Work out the finished part from the listing and answer in its coordinate system (mm). Face numbers are marked on the shaded views. A direction names the side the tool comes from. Give positions to 0.01 mm unless a question says otherwise; leave off trailing zeros. Write each loop counter-clockwise with the first axis right and the second up, starting at its lowest first coordinate (ties: lowest second). Pieces come first, ordered by that corner, then holes.
1) Given pin 1 Ø2 at (y, z) = (-7, 47) entering from +X; pin 2 Ø12 at (x, y) = (37, 0) entering from -Z; pin 3 Ø8.5 at (x, y) = (130.58, -8.08) entering from +Z; pin 4 Ø6 at (y, z) = (-6, 15) entering from -X, each flat-ended and moving along its own axis, determine where each tip first touches the part or whether it passes through.
2) Find section D-D (x = -1.5). Determine the outline of the cut face in (y, z), plus the area to 3 significant figures.
3) A tool of negligible diameter and unlimited length cuts with its end or side. For the marked faces 5, 6, 7 and 8, from which of +Z, -Z, +X, -X, +Y, -Y can it reach the whole face along a straight path? Write none if from no direction.
4) Find section C-C (x = 62). Determine the outline of the cut face in (y, z), plus the area to 3 significant figures.
5) Determine the mould class of the marked faces 1, 2, 3 and 4 for opening direction Z: pulls with the +Z half, pulls with the -Z half, needs draft (parallel to the pull), parting line crosses it, or undercut.
6) Find section A-A (z = 15.5). Determine the outline of the cut face in (x, y).
7) Find section B-B (y = -14). Determine the outline of the cut face in (x, z).
8) Straight lines are drawn through the part: probe 1 along X at (y, z) = (-4, 19.5); probe 2 along Z at (x, y) = (68.5, 2.5); probe 3 along Z at (x, y) = (133.5, 4). For each, find the intervals that lie inside material, in ascending order.
```python
from build123d import *

# Parameters (mm, degrees)
SKETCH1_R           = 3.175
BOSS_EXTRUDE1_DEPTH = 11.43
SKETCH2_W           = 161.464261653
SKETCH2_H           = 32
BOSS_EXTRUDE2_DEPTH = 12.7
SKETCH5_R           = 3.175
BOSS_EXTRUDE3_DEPTH = 11.43
SKETCH6_W           = 77
SKETCH6_H           = 11.5
CUT_EXTRUDE1_DEPTH  = 7.5
BOSS_EXTRUDE4_DEPTH = 19.05
CUT_EXTRUDE3_DEPTH  = 30.48
BOSS_EXTRUDE5_DEPTH = 25.4
SKETCH7_W           = 12
SKETCH7_H           = 11.5
CUT_EXTRUDE4_DEPTH  = 50.8
SKETCH7_5_W         = 12
SKETCH7_5_H         = 11.5
CUT_EXTRUDE5_DEPTH  = 50.8


with BuildPart() as part:
    # Sketch1 → Boss-Extrude1 (new body)
    with BuildSketch(Plane.XY):
        with BuildLine():
            Line((-47.217391304, 7.923913043), (130.582608696, 7.923913043))
            ThreePointArc((130.582608696, 7.923913043), (146.582608696, -8.076086957), (130.582608696, -24.076086957))
            Line((130.582608696, -24.076086957), (-47.217391304, -24.076086957))
            ThreePointArc((-47.217391304, -24.076086957), (-63.217391304, -8.076086957), (-47.217391304, 7.923913043))
        make_face()
        with Locations((-47.217391304, -8.076086957)):
            Circle(SKETCH1_R, mode=Mode.SUBTRACT)
        with Locations((130.582608696, -8.076086957)):
            Circle(SKETCH1_R, mode=Mode.SUBTRACT)
    extrude(amount=BOSS_EXTRUDE1_DEPTH)

    # Sketch2 → Boss-Extrude2 (add)
    with BuildSketch(Plane.XY.offset(11.43)):
        with Locations((41.59547787, -8.076086957)):
            Rectangle(SKETCH2_W, SKETCH2_H)
    extrude(amount=BOSS_EXTRUDE2_DEPTH)

    # Sketch5 → Boss-Extrude3 (add)
    with BuildSketch(Plane.XY.offset(24.13)):
        with BuildLine():
            Line((-47.217391304, 7.923913043), (130.582608696, 7.923913043))
            ThreePointArc((130.582608696, 7.923913043), (146.582608696, -8.076086957), (130.582608696, -24.076086957))
            Line((130.582608696, -24.076086957), (-47.217391304, -24.076086957))
            ThreePointArc((-47.217391304, -24.076086957), (-63.217391304, -8.076086957), (-47.217391304, 7.923913043))
        make_face()
        with Locations((-47.217391304, -8.076086957)):
            Circle(SKETCH5_R, mode=Mode.SUBTRACT)
        with Locations((130.582608696, -8.076086957)):
            Circle(SKETCH5_R, mode=Mode.SUBTRACT)
    extrude(amount=BOSS_EXTRUDE3_DEPTH)

    # Sketch6 → Cut-Extrude1 (cut)
    with BuildSketch(Plane(origin=(0, 7.923913043, 0), x_dir=(1, 0, 0), z_dir=(0, 1, 0))):
        with Locations((41.682608696, -17.78)):
            Rectangle(SKETCH6_W, SKETCH6_H)
    extrude(amount=-CUT_EXTRUDE1_DEPTH, mode=Mode.SUBTRACT)

    # Sketch10 → Boss-Extrude4 (add)
    with BuildSketch(Plane.XY.offset(35.56)):
        with BuildLine():
            Line((-34.517391304, -20.776086957), (-57.377391304, -20.776086957))
            ThreePointArc((-57.377391304, -20.776086957), (-59.173442529, -20.032138181), (-59.917391304, -18.236086957))
            Line((-59.917391304, -18.236086957), (-59.917391304, 2.083913043))
            ThreePointArc((-59.917391304, 2.083913043), (-59.173442529, 3.879964268), (-57.377391304, 4.623913043))
            Line((-57.377391304, 4.623913043), (-34.517391304, 4.623913043))
            Line((-34.517391304, 4.623913043), (-21.817391304, 4.623913043))
            Line((-21.817391304, 4.623913043), (-21.817391304, -20.776086957))
            Line((-21.817391304, -20.776086957), (-34.517391304, -20.776086957))
        make_face()
    extrude(amount=BOSS_EXTRUDE4_DEPTH)

    # Sketch14 → Cut-Extrude3 (cut)
    with BuildSketch(Plane(origin=(0, 4.623913043, 0), x_dir=(1, 0, 0), z_dir=(0, 1, 0))):
        with BuildLine():
            Line((-59.917391304, -35.56), (-29.183391304, -35.56))
            ThreePointArc((-29.183391304, -35.56), (-29.434604535, -44.304535578), (-35.79555952, -50.310221405))
            Line((-35.79555952, -50.310221405), (-59.917391304, -50.310221405))
            Line((-59.917391304, -50.310221405), (-59.917391304, -35.56))
        make_face()
    extrude(amount=-CUT_EXTRUDE3_DEPTH, mode=Mode.SUBTRACT)

    # Sketch15 → Boss-Extrude5 (add)
    with BuildSketch(Plane.XZ.offset(20.776086957)):
        Polygon((-21.817391304, 35.56), (5.46367495, 35.56), (-21.817391304, 54.61), align=None)
    extrude(amount=-BOSS_EXTRUDE5_DEPTH)

    # Sketch7 → Cut-Extrude4 (cut)
    with BuildSketch(Plane(origin=(0, 0.423913043, 0), x_dir=(1, 0, 0), z_dir=(0, 1, 0))):
        with Locations((74.182608696, -17.78)):
            Rectangle(SKETCH7_W, SKETCH7_H)
    extrude(amount=-CUT_EXTRUDE4_DEPTH, mode=Mode.SUBTRACT)

    # Sketch7<5> → Cut-Extrude5 (cut)
    with BuildSketch(Plane(origin=(0, 0.423913043, 0), x_dir=(1, 0, 0), z_dir=(0, 1, 0))):
        with Locations((9.182608696, -17.78)):
            Rectangle(SKETCH7_5_W, SKETCH7_5_H)
    extrude(amount=-CUT_EXTRUDE5_DEPTH, mode=Mode.SUBTRACT)


solid = part.part
```
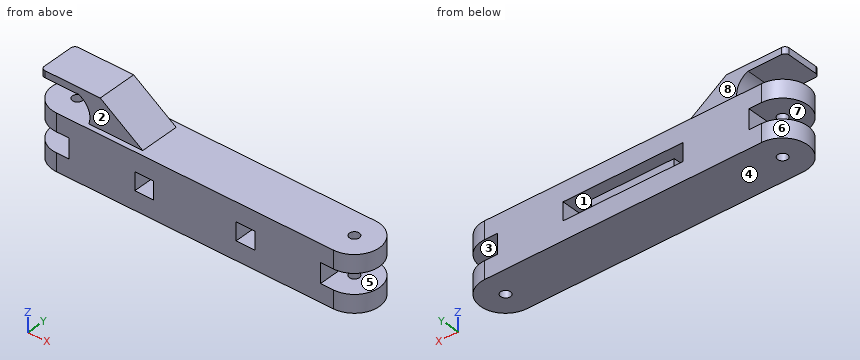
Results:
1. pin 1: stops at x = -9.49
1. pin 2: stops at z = 0
1. pin 3: stops at z = 35.56
1. pin 4: stops at x = -39.14
2. outline: (-24.08, 0) - (7.92, 0) - (7.92, 35.56) - (4.62, 35.56) - (4.62, 40.42) - (-20.78, 40.42) - (-20.78, 35.56) - (-24.08, 35.56) - close
2. area: 1,260 mm2
3. face 5: +X, +Y, -Y
3. face 6: -Z, -X
3. face 7: -X, +Y, -Y
3. face 8: +Z, +X, -X, +Y
4. outline: (-24.08, 0) - (7.92, 0) - (7.92, 12.03) - (0.42, 12.03) - (0.42, 23.53) - (7.92, 23.53) - (7.92, 35.56) - (-24.08, 35.56) - close
4. area: 1,050 mm2
5. face 1: undercut
5. face 2: needs draft
5. face 3: undercut
5. face 4: pulls with the -Z half
6. outline: (-39.14, -24.08) - (3.18, -24.08) - (3.18, 7.92) - (-39.14, 7.92) - close; (15.18, -24.08) - (68.18, -24.08) - (68.18, 0.42) - (15.18, 0.42) - close; (80.18, -24.08) - (122.33, -24.08) - (122.33, 7.92) - (80.18, 7.92) - close
7. outline: (-62.08, 0) - (145.45, 0) - (145.45, 11.43) - (122.33, 11.43) - (122.33, 24.13) - (145.45, 24.13) - (145.45, 35.56) - (5.46, 35.56) - (-21.82, 54.61) - (-59.92, 54.61) - (-59.92, 50.31) - (-35.8, 50.31) arc R11.43 cw to (-29.18, 35.56) - (-62.08, 35.56) - (-62.08, 24.13) - (-39.14, 24.13) - (-39.14, 11.43) - (-62.08, 11.43) - close; hole (3.18, 12.03) - (15.18, 12.03) - (15.18, 23.53) - (3.18, 23.53) - close; hole (68.18, 12.03) - (80.18, 12.03) - (80.18, 23.53) - (68.18, 23.53) - close
8. probe 1: x = -39.14 to 3.18, 15.18 to 68.18, 80.18 to 122.33
8. probe 2: z = 0 to 12.03, 23.53 to 35.56
8. probe 3: z = 0 to 11.43, 24.13 to 35.56
